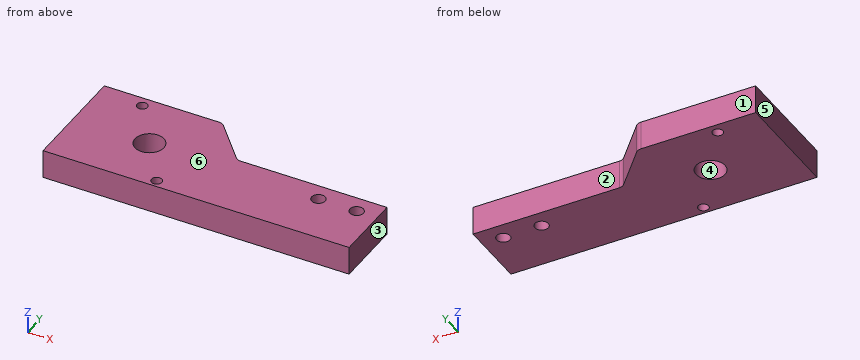
```python
from build123d import *

# Parameters (mm, degrees)
SKETCH1_W                 = 101.6
SKETCH1_H                 = 50.8
BOSS_EXTRUDE1_DEPTH       = 9.525
SKETCH6_R                 = 4.8
CUT_EXTRUDE1_DEPTH        = 58.589283942
TAP_DRILL_FOR_8_32_TAP1_D = 3.4544
F_8_CLEARANCE_HOLE1_D     = 4.4958
SKETCH10_W                = 101.6
SKETCH10_H                = 37.138907791
CUT_EXTRUDE2_DEPTH        = 58.589283942
CUT_EXTRUDE3_DEPTH        = 58.589283942
FILLET1_R                 = 2.54


with BuildPart() as part:
    # Sketch1 → Boss-Extrude1 (new body)
    with BuildSketch(Plane.XY):
        Rectangle(SKETCH1_W, SKETCH1_H)
    extrude(amount=BOSS_EXTRUDE1_DEPTH)

    # Sketch6 → Cut-Extrude1 (cut, through all)
    with BuildSketch(Plane.XY):
        with Locations(Location((-25.4, 6.35, 0), (0, 0, 180))):
            Circle(SKETCH6_R)
    extrude(amount=CUT_EXTRUDE1_DEPTH, mode=Mode.SUBTRACT)

    # Tap Drill for #8-32 Tap1 (through all)
    with Locations(Plane.XY.offset(9.525)):
        with Locations((-14.502047709, -9.213888841), (-36.297952291, 21.913888841)):
            Hole(TAP_DRILL_FOR_8_32_TAP1_D / 2)

    # #8 Clearance Hole1 (through all)
    with Locations(Plane.XY.offset(9.525)):
        with Locations((31.231814057, 5.34348178), (43.931814057, 5.34348178)):
            Hole(F_8_CLEARANCE_HOLE1_D / 2)

    # Sketch10 → Cut-Extrude2 (cut, through all)
    with BuildSketch(Plane.XY.offset(9.525)):
        with Locations((0, -30.370972115)):
            Rectangle(SKETCH10_W, SKETCH10_H)
    extrude(amount=-CUT_EXTRUDE2_DEPTH, mode=Mode.SUBTRACT)

    # Sketch11 → Cut-Extrude3 (cut, through all)
    with BuildSketch(Plane.XY.offset(9.525)):
        Polygon((50.8, 11.193885079), (1.096095255, 11.193885079), (-11.576646979, 25.4), (50.8, 25.4), align=None)
    extrude(amount=-CUT_EXTRUDE3_DEPTH, mode=Mode.SUBTRACT)

    # Fillet1
    fillet1_edges = [part.edges().sort_by_distance(p)[0] for p in [
        (1.096095255, 11.193885079, 4.7625),
        (-11.576646979, 25.4, 4.7625),
    ]]
    fillet(fillet1_edges, radius=FILLET1_R)


solid = part.part
```
The listing builds one solid part. Answer for the finished solid, in the listing's coordinates (mm). Face numbers are marked on the shaded views. A direction names the side the tool comes from. Coordinates: 2 decimals unless noted, no trailing zeros. Order: outer loops, then holes, each group sorted by start corner. A loop starts at its lowest first (then second) coordinate and runs counter-clockwise, first axis right, second up. Notation, with made-up numbers: M 37,34 L 49,34 A22 ccw 49,72 Z; hole C 42,67.25 d7. An arc over 180 degrees is marked long. Answer as a JSON object with one key per item and string values. Group by question number.
1. Determine the mould class of the marked faces 3, 4, 5 and 6 for opening direction X: released by +X, released by -X, zero draft, split by the parting line, or undercut.
2. Section A-A on x = -25.4 is taken. Write down the section's boundary in (y, z) (3 decimals).
3. Section D-D on x = 17 is taken. Write down the section's boundary in (y, z) (3 decimals), then the cut area to 3 significant figures.
4. A tool of negligible diameter and unlimited length cuts with its end or side. For the marked faces 1 and 2, from which of +Z, -Z, +X, -X, +Y, -Y can it reach the whole face along a straight path? Write none if from no direction.
5. Section B-B on y = 6.35 is taken. Write down the section's boundary in (x, z) (3 decimals).
6. Straight lines are drawn through the part: line 1 (X direction, y = 21, z = 8); line 2 (Y direction, x = -16, z = 5.75); line 3 (X direction, y = 9, z = 0.75). For each, find the intervals that lie inside material, in ascending order.
7. Flat-ended cylindrical pins translate along their axes: P1, Ø2, axis at y = 19, z = 8, coming from the +X side; P2, Ø10, axis at x = -26, y = 5, coming from the +Z side (3 decimals); P3, Ø3, axis at x = 19.5, z = 3, coming from the +Y side. Find the tip coordinate at first contact, or state that the pin passes through.
8. Section C-C on z = 1.75 is taken. Write down the section's boundary in (x, y), then the cut area to 3 significant figures.
Values follow:
{
 "1": {"face 3": "released by +X", "face 4": "undercut", "face 5": "released by -X", "face 6": "zero draft"},
 "2": {"outline": "M -11.802,0 L 1.55,0 L 1.55,9.525 L -11.802,9.525 Z; M 11.15,0 L 25.4,0 L 25.4,9.525 L 11.15,9.525 Z"},
 "3": {"outline": "M -11.802,0 L 11.194,0 L 11.194,9.525 L -11.802,9.525 Z", "area": "219 mm2"},
 "4": {"face 1": "+Z, -Z, +X, -X, +Y", "face 2": "+Z, -Z, +X, +Y"},
 "5": {"outline": "M -50.8,0 L -30.2,0 L -30.2,9.525 L -50.8,9.525 Z; M -20.6,0 L 29.222,0 L 29.222,9.525 L -20.6,9.525 Z; M 33.242,0 L 41.922,0 L 41.922,9.525 L 33.242,9.525 Z; M 45.942,0 L 50.8,0 L 50.8,9.525 L 45.942,9.525 Z"},
 "6": {"line 1": "-50.8 to -37.76, -34.83 to -7.65", "line 2": "-11.8 to -10.07, -8.35 to 25.4", "line 3": "-50.8 to -29.4, -21.4 to 50.8"},
 "7": {"P1": "x = -4.98", "P2": "z = 9.525", "P3": "y = 11.19"},
 "8": {"outline": "M -50.8,-11.8 L 50.8,-11.8 L 50.8,11.19 L 2.23,11.19 A2.54 cw 0.34,12.04 L -10.82,24.55 A2.54 ccw -12.71,25.4 L -50.8,25.4 Z; hole C -36.3,21.91 d3.45; hole C -25.4,6.35 d9.6; hole C -14.5,-9.21 d3.45; hole C 31.23,5.34 d4.5; hole C 43.93,5.34 d4.5", "area": "2,860 mm2"}
}
